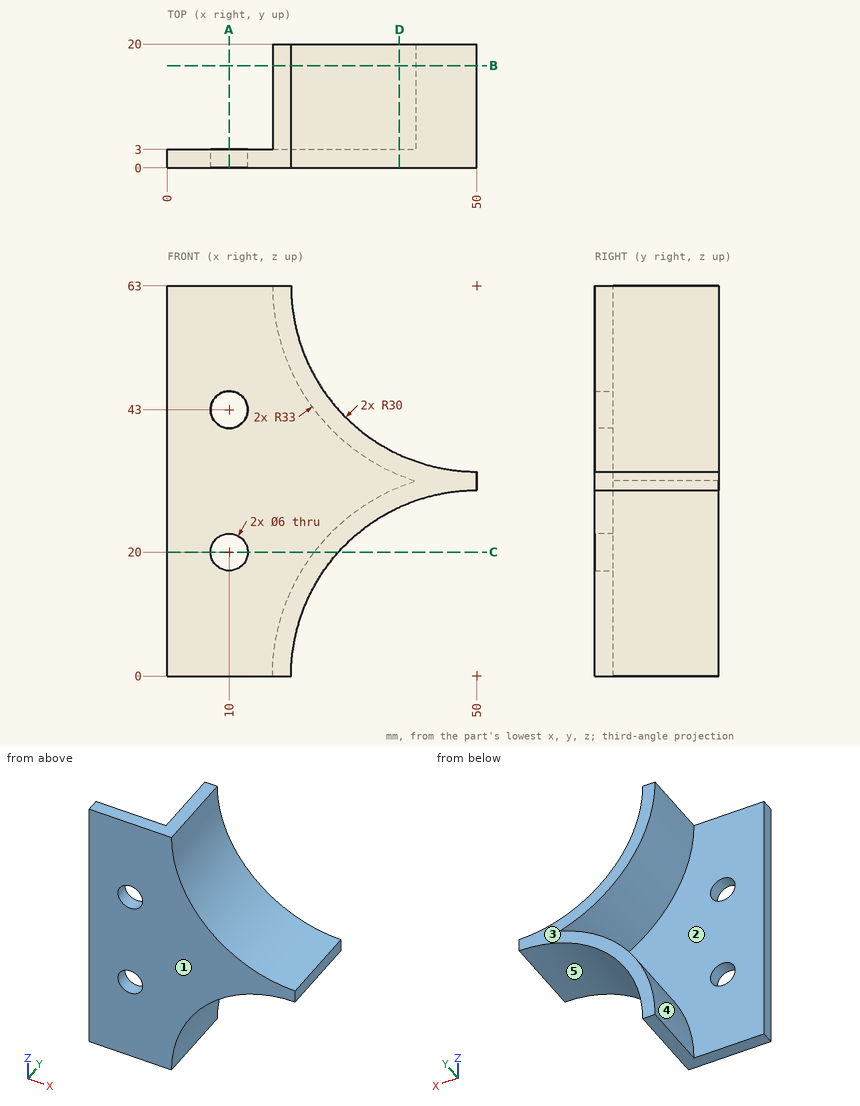
Design review of the part shown in the three views and the two pictorial views. Dimensions are in mm from the part's minimum x, y and z. A direction names the side the tool comes from. Round coordinates to 2 decimals unless told otherwise and drop trailing zeros. Loops run counter-clockwise (first coordinate to the right, second up) from the corner with the lowest first, then second, coordinate; pieces in that order, holes last. Notation, with made-up numbers: (61.25, -36) -> (115.25, -36) arc R31 ccw to (115.25, -6) -> close; hole circle Ø6 at (-0.5, -8). An arc over 180 degrees is marked (long way). Use one line per item in the form item = value. Start each with the question number.
Q1. We need section D-D on x = 37.5. Give the boundary of the cut face in (y, z), then the cut area to 3 significant figures.
Q2. We need section B-B on y = 16.5. Give the boundary of the cut face in (x, z).
Q3. Draft analysis for pull direction Z (two halves, no side actions). For the marked faces 3, 4 and 5, state which applies: +Z half, -Z half, draft (parallel to the pull), parting line (faces both ways), or undercut.
Q4. Machinability: for the marked faces 1 and 2, which of the approach directions +Z, -Z, +X, -X, +Y, -Y give a long, thin tool a straight path to every point of the face, cutting with its end or side? Answer none if there is none.
Q5. We need section C-C on z = 20. Give the boundary of the cut face in (x, y).
Q6. We need section A-A on x = 10. Give the boundary of the cut face in (y, z), then the cut area to 3 significant figures.
Q7. For pin 1 Ø5 at (x, z) = (10, 20) entering from +Y; pin 2 Ø2 at (y, z) = (8.5, 25) entering from -X; pin 3 Ø12 at (x, z) = (16, 35) entering from +Y; pin 4 Ø1 at (x, y) = (30.5, 17.5) entering from +Z, all flat-tipped, find the tip position at first contact; note any pin that passes through.
Q8. Wall thickness on line 1 along Y through (x, z) = (34.5, 32.5); line 2 along Z through (x, y) = (29, 15.75); line 3 along X through (y, z) = (1.9, 20): over which ranges is each line inside the solid? List them lowest first. Write a range as [from, to].
Calculated:
q1.outline = (0, 27.27) -> (20, 27.27) -> (20, 30.54) -> (3, 30.54) -> (3, 32.46) -> (20, 32.46) -> (20, 35.73) -> (0, 35.73) -> close
q1.area = 137 mm²
q2.outline = (17, 0) -> (20, 0) arc R30 cw to (50, 30) -> (50, 33) arc R30 cw to (20, 63) -> (17, 63) arc R33 ccw to (40.16, 31.5) arc R33 ccw to start
q3.face_3 = draft
q3.face_4 = undercut
q3.face_5 = -Z half
q4.face_1 = +Z, -Z, +X, -X, -Y
q4.face_2 = -X, +Y
q5.outline = (0, 0) -> (7, 0) -> (7, 3) -> (0, 3) -> close; (13, 0) -> (27.64, 0) -> (27.64, 20) -> (23.75, 20) -> (23.75, 3) -> (13, 3) -> close
q6.outline = (0, 0) -> (3, 0) -> (3, 17) -> (0, 17) -> close; (0, 23) -> (3, 23) -> (3, 40) -> (0, 40) -> close; (0, 46) -> (3, 46) -> (3, 63) -> (0, 63) -> close
q6.area = 153 mm²
q7.pin_1 = through
q7.pin_2 = 27.35
q7.pin_3 = 3
q7.pin_4 = 40.64
q8.line_1 = [0, 3]
q8.line_2 = [21.42, 25.46], [37.54, 41.58]
q8.line_3 = [0, 7], [13, 27.64]
